```python
from build123d import *

# Parameters (mm, degrees)
INNERC_SIZE = 0.4
OUTERC_SIZE = 0.1


with BuildPart() as part:
    # BodyS → Body (revolve)
    with BuildSketch(Plane.XY):
        Polygon((6, -3.25), (6, 3.25), (9, 3.25), (9, 4.25), (4, 4.25), (4, 0.25), (3.5, 0.25), (3.5, -0.25), (4, -0.25), (4, -4.25), (9, -4.25), (9, -3.25), align=None)
    revolve(axis=Axis((0, 4.25, 0), (0, -1, 0)))

    # InnerC
    innerc_edges = [part.edges().sort_by_distance(p)[0] for p in [
        (-4, -4.25, 0),
        (-4, 4.25, 0),
    ]]
    chamfer(innerc_edges, length=INNERC_SIZE)

    # OuterC
    outerc_edges = [part.edges().sort_by_distance(p)[0] for p in [
        (-9, 4.25, 0),
        (-9, 3.25, 0),
        (-9, -3.25, 0),
        (-9, -4.25, 0),
    ]]
    chamfer(outerc_edges, length=OUTERC_SIZE)


solid = part.part
```
Part model, mm, in its own coordinate system. A direction names the side the tool comes from. Coordinates: 2 decimals unless noted, no trailing zeros. Write each loop counter-clockwise with the first axis right and the second up, starting at its lowest first coordinate (ties: lowest second). Pieces come first, ordered by that corner, then holes.
Item 1: Pin check, flat tips, straight feed: pin 1 (1 mm diameter, centred on y = -1, z = 4, fed in from +X); pin 2 (5 mm diameter, centred on y = 0, z = -2.5, fed in from -X); pin 3 (3 mm diameter, centred on x = 3, y = -0.5, fed in from +Z); pin 4 (9 mm diameter, centred on x = -0.5, z = 1, fed in from -Y). Stop position of each tip, or through.
Item 2: Probe line 1 (Z direction, x = 0, y = 0.1); line 2 (Z direction, x = 0, y = 1.3); line 3 (Y direction, x = 1, z = 7.5). List the from-to ranges inside material, lowest first.
Item 3: Slice it at A-A (y = 1.25). Write the cut outline in (x, z).
Item 4: Mould opens along Y. For faces 4 (the face through (2.1, -4.25, 4.1)), 5 (the face through (-1.172, 3.756, 8.923)), 6 (the face through (-6, 0, 0)) say: released by +Y, released by -Y, zero draft, split by the parting line, or undercut.
Item 5: Which spindle directions (+Z, -Z, +X, -X, +Y, -Y) get a long thin tool onto all of the face, cutting with end or side? Do faces 1 (the face through (2, -3.25, -6)), 2 (the face through (-0.867, -2.075, -3.905)), 3 (the face through (-0.867, 2.025, -3.905)). Say none if no direction does.
Results found:
1. pin 1: stops at x = 4.87
1. pin 2: stops at x = -6
1. pin 3: stops at z = 5.81
1. pin 4: stops at y = -4.25
2. line 1: z = -6 to -3.5, 3.5 to 6
2. line 2: z = -6 to -4, 4 to 6
2. line 3: y = -4.25 to -3.25, 3.25 to 4.25
3. outline: circle Ø12 at (0, 0); hole circle Ø8 at (0, 0)
4. face 4: released by -Y
4. face 5: zero draft
4. face 6: undercut
5. face 1: none
5. face 2: -Y
5. face 3: +Y
